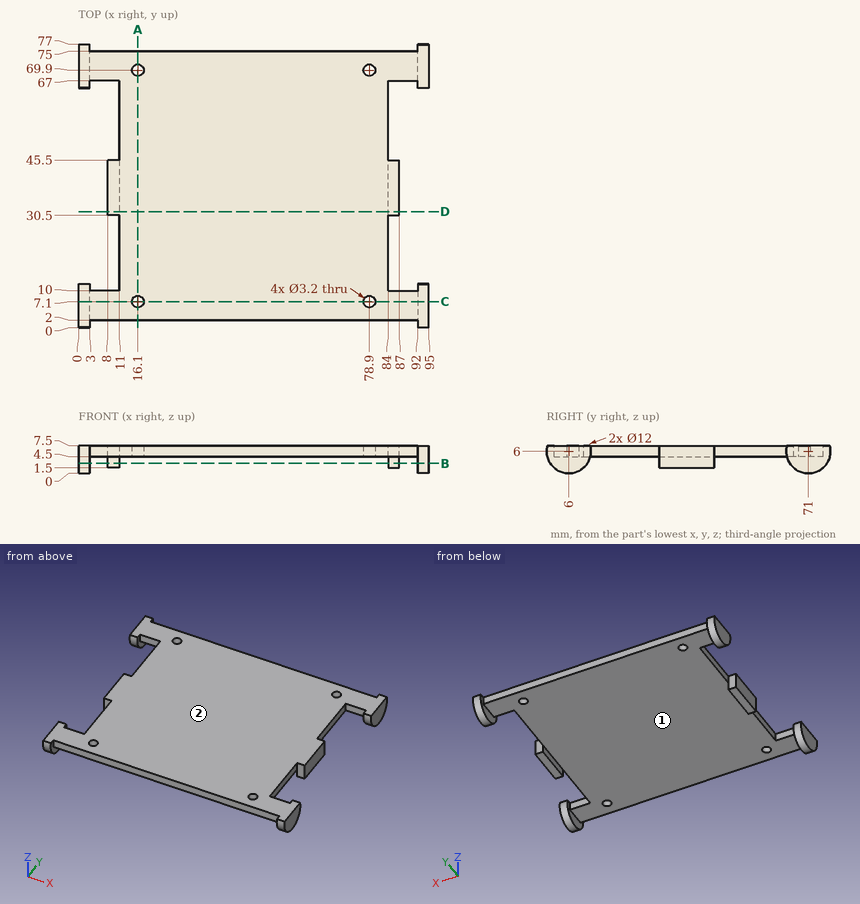
Could you check a few things on this drawing? It's one solid part, dimensions in mm from its lowest x, y, z. Give positions to 0.01 mm unless a question says otherwise; leave off trailing zeros. Order: outer loops, then holes, each group sorted by start corner. A loop starts at its lowest first (then second) coordinate and runs counter-clockwise, first axis right, second up. Notation, with made-up numbers: (47.5, 56.5) - (91.5, 56.5) arc R16 ccw to (91.5, 64.5) - close; hole circle Ø3 at (13.5, 66.25). An arc over 180 degrees is marked (long way). One line per item, written item: value. Start each with the question number.
1. Imagine slicing it at C-C on y = 7.1. List the corners of the cut face in (x, z) for me, plus the area to 3 significant figures.
2. Imagine slicing it at D-D on y = 31.5. List the corners of the cut face in (x, z) for me, plus the area to 3 significant figures.
3. For P1, Ø2, axis at y = 24, z = 5, coming from the +X side; P2, Ø5, axis at x = 78.9, y = 7.1, coming from the -Z side; P3, Ø2, axis at y = 32.5, z = 2, coming from the +X side, each with a flat end and sliding along its axis, tell me the tip position at first contact or that it passes through.
4. Thinking about a two-plate mould opening in Z: for the marked faces 1 and 2, which applies, +Z half, -Z half, draft (parallel to the pull), parting line (faces both ways), or undercut?
5. Imagine slicing it at A-A on x = 16.1. List the corners of the cut face in (y, z) for me.
6. Imagine slicing it at B-B on z = 2.75. List the corners of the cut face in (x, y) for me, plus the area to 3 significant figures.
7. If I drill on probe 1 along X at (y, z) = (7.1, 5.8); probe 2 along Y at (x, z) = (78.9, 5.55); probe 3 along Z at (x, y) = (52.5, 23), over which ranges is the centre line in solid material (lowest first)?
Values:
1. outline: (0, 0.1) - (3, 0.1) - (3, 4.5) - (14.5, 4.5) - (14.5, 7.5) - (0, 7.5) - close; (17.7, 4.5) - (77.3, 4.5) - (77.3, 7.5) - (17.7, 7.5) - close; (80.5, 4.5) - (92, 4.5) - (92, 0.1) - (95, 0.1) - (95, 7.5) - (80.5, 7.5) - close
1. area: 292 mm²
2. outline: (8, 1.5) - (11, 1.5) - (11, 4.5) - (84, 4.5) - (84, 1.5) - (87, 1.5) - (87, 7.5) - (8, 7.5) - close
2. area: 255 mm²
3. P1: x = 84
3. P2: z = 4.5
3. P3: x = 87
4. face 1: -Z half
4. face 2: +Z half
5. outline: (2, 4.5) - (5.5, 4.5) - (5.5, 7.5) - (2, 7.5) - close; (8.7, 4.5) - (68.3, 4.5) - (68.3, 7.5) - (8.7, 7.5) - close; (71.5, 4.5) - (75, 4.5) - (75, 7.5) - (71.5, 7.5) - close
6. outline: (0, 0.96) - (3, 0.96) - (3, 11.04) - (0, 11.04) - close; (0, 65.96) - (3, 65.96) - (3, 76.04) - (0, 76.04) - close; (8, 30.5) - (11, 30.5) - (11, 45.5) - (8, 45.5) - close; (84, 30.5) - (87, 30.5) - (87, 45.5) - (84, 45.5) - close; (92, 0.96) - (95, 0.96) - (95, 11.04) - (92, 11.04) - close; (92, 65.96) - (95, 65.96) - (95, 76.04) - (92, 76.04) - close
6. area: 211 mm²
7. probe 1: 0 to 14.5, 17.7 to 77.3, 80.5 to 95
7. probe 2: 2 to 5.5, 8.7 to 68.3, 71.5 to 75
7. probe 3: 4.5 to 7.5
